Work out the finished part from the listing and answer in its coordinate system (mm). A direction names the side the tool comes from. Give positions to 0.01 mm unless a question says otherwise; leave off trailing zeros. Write each loop counter-clockwise with the first axis right and the second up, starting at its lowest first coordinate (ties: lowest second). Pieces come first, ordered by that corner, then holes. Notation, with made-up numbers: (-29, 52) - (23, 52) arc R24 ccw to (23, 75) - close; hole circle Ø8 at (57.5, -12.5). An arc over 180 degrees is marked (long way). Write each question's results on one line, items separated by ' | '. Start each with the question number.
from build123d import *

# Parameters (mm, degrees)
F1_DEPTH = 10.922
F0_W     = 10.922
F0_H     = 33.528
F2_DEPTH = 50.8
F3_DEPTH = 60.198
F5_DEPTH = 10.923
F7_DEPTH = 10.923


with BuildPart() as f1:
    # F0 (on Front) → F1 (new body)
    with BuildSketch(Plane.XZ):
        Polygon((-46.228, -22.225), (-6.35, 11.303), (-46.228, 11.303), align=None)
    extrude(amount=F1_DEPTH)

    # F0 (on Front) → F2 (join)
    with BuildSketch(Plane.XZ):
        with Locations((-51.689, -5.461)):
            Rectangle(F0_W, F0_H)
    extrude(amount=F2_DEPTH)

    # F0 (on Front) → F3 (join)
    with BuildSketch(Plane.XZ):
        Polygon((57.15, 11.303), (57.15, 22.225), (-57.15, 22.225), (-57.15, 11.303), (-46.228, 11.303), (-6.35, 11.303), align=None)
    extrude(amount=F3_DEPTH)

    # F4 (on face) → F5 (cut, through all)
    with BuildSketch(Plane(origin=(0, 0, 11.303), x_dir=(1, 0, 0), z_dir=(0, 0, -1))):
        with BuildLine():
            ThreePointArc((38.1, 11.176), (43.667759, 13.482241), (45.974, 19.05))
            ThreePointArc((45.974, 19.05), (32.532241, 24.617759), (38.1, 11.176))
        make_face()
        Polygon((57.15, 60.198), (-25.4, 60.198), (57.15, 38.078794), align=None)
    extrude(amount=-F5_DEPTH, mode=Mode.SUBTRACT)

    # F6 (on face) → F7 (cut, through all)
    with BuildSketch(Plane.YZ.offset(-46.228)):
        Polygon((-50.8, -5.461), (-50.8, -22.225), (-22.098, -22.225), align=None)
    extrude(amount=-F7_DEPTH, mode=Mode.SUBTRACT)


solid = f1.part
Q1. A cutting plane is placed at D-D, the plane z = 6.5. Write down the section's boundary in (x, y).
Q2. Consider L1, parallel to X at y = -19.05, z = 17; L2, parallel to Z at x = 13, y = -12 (3 decimals); L3, parallel to X at y = -17.5, z = -6. Determine where each line is inside the solid, lowest interval first.
Q3. A cutting plane is placed at C-C, the plane y = -6.5. Write down the section's boundary in (x, z) (3 decimals).
Q4. Given pin 1 (1.5 mm diameter, centred on x = -18.5, y = -50.5, fed in from -Z); pin 2 (8.5 mm diameter, centred on x = -51.5, z = -1, fed in from -Y); pin 3 (3 mm diameter, centred on y = -32, z = -10, fed in from +X); pin 4 (18 mm diameter, centred on x = 38.1, y = -19.05, fed in from +Z) (3 decimals), each flat-ended and moving along its own axis, determine where each tip first touches the part or whether it passes through.
Q5. A cutting plane is placed at A-A, the plane x = 34.5. Write down the section's boundary in (y, z) (3 decimals), and give its area (3 significant figures).
Q6. A tool of negligible diameter and unlimited length cuts with its end or side. For faces 1 (the flat face through (-46.228, -31, -2)), 2 (the flat face through (-52, -50.8, 3)), 3 (the flat face through (15.297, -49.293, 16.688)), from which of +Z, -Z, +X, -X, +Y, -Y can it reach the whole face along a straight path? Write none if from no direction.
Q7. A cutting plane is placed at B-B, the plane y = -14. Write down the section's boundary in (x, z) (3 decimals), and give its area (3 significant figures).
Result:
1) outline: (-57.15, -50.8) - (-46.23, -50.8) - (-46.23, -10.92) - (-12.06, -10.92) - (-12.06, 0) - (-57.15, 0) - close
2) L1: x = -57.15 to 30.23, 45.97 to 57.15 | L2: z = 11.303 to 22.225 | L3: x = -57.15 to -46.23
3) outline: (-57.15, -22.225) - (-46.228, -22.225) - (-6.35, 11.303) - (57.15, 11.303) - (57.15, 22.225) - (-57.15, 22.225) - close
4) pin 1: stops at z = 11.3 | pin 2: stops at y = -50.8 | pin 3: stops at x = -46.23 | pin 4: stops at z = 22.225
5) outline: (-44.148, 11.303) - (-26.053, 11.303) - (-26.053, 22.225) - (-44.148, 22.225) - close; (-12.047, 11.303) - (0, 11.303) - (0, 22.225) - (-12.047, 22.225) - close | area: 329 mm2
6) face 1: -Z, +X, -Y | face 2: -Z, +X, -X, -Y | face 3: +Z, -Z, +X, -Y
7) outline: (-57.15, -22.225) - (-46.228, -22.225) - (-46.228, 11.303) - (32.059, 11.303) - (32.059, 22.225) - (-57.15, 22.225) - close; (44.141, 11.303) - (57.15, 11.303) - (57.15, 22.225) - (44.141, 22.225) - close | area: 1,480 mm2
